Model file for the job. Use its own axes, mm. A direction names the side the tool comes from. Coordinates: 2 decimals unless noted, no trailing zeros. Order: outer loops, then holes, each group sorted by start corner. A loop starts at its lowest first (then second) coordinate and runs counter-clockwise, first axis right, second up.
from build123d import *

# Parameters (mm, degrees)
F1_DEPTH      = 152.4
F1_DEPTH_BACK = 152.4
F2_W          = 381.0055409819
F2_H          = 19.05
F2_W_2        = 381
F3_DEPTH      = 6.096
F4_W          = 381.0055409819
F4_H          = 19.05
F4_W_2        = 381
F5_DEPTH      = 6.096


# Not quite as in the source:
# - ends of sketch curves that miss each other by under 0.0002 mm in the source are joined


with BuildPart() as f1:
    # F0 (on Front) → F1 (new body, two sides)
    with BuildSketch(Plane.XZ) as f1_sk:
        Polygon((-533.4, -382.5126007106), (-381, -382.5126007106), (-381, -378.4719215088), (0, -378.4719215088), (0, -359.4219215088), (-381, -359.4219215088), (-381, -356.2469204928), (-381, -12.157774965), (-381, -8.982775981), (0.0055409819, -8.982775981), (0.0055409819, 10.067224019), (-381, 10.067224019), (-381, 13.242225035), (-381, 355.2765448173), (-381, 358.4515458333), (0.0055409819, 358.4515458333), (0.0055409819, 377.5015458333), (-381, 377.5015458333), (-381, 380.6765448173), (-533.4, 380.6765468493), align=None)
    extrude(amount=F1_DEPTH)
    extrude(f1_sk.sketch, amount=-F1_DEPTH_BACK)

    # F2 (on face) → F3 (cut)
    with BuildSketch(Plane(origin=(0, 152.4, 0), x_dir=(-1, 0, 0), z_dir=(0, 1, 0))):
        with Locations((190.4972295091, 367.9765458333)):
            Rectangle(F2_W, F2_H)
        with Locations((190.4972295091, 0.542224019)):
            Rectangle(F2_W, F2_H)
        with Locations((190.5, -368.9469215088)):
            Rectangle(F2_W_2, F2_H)
    extrude(amount=-F3_DEPTH, mode=Mode.SUBTRACT)

    # F4 (on face) → F5 (cut)
    with BuildSketch(Plane.XZ.offset(152.4)):
        with Locations((-190.4972295091, 0.542224019)):
            Rectangle(F4_W, F4_H)
        with Locations((-190.4972295091, 367.9765458333)):
            Rectangle(F4_W, F4_H)
        with Locations((-190.5, -368.9469215088)):
            Rectangle(F4_W_2, F4_H)
    extrude(amount=-F5_DEPTH, mode=Mode.SUBTRACT)


solid = f1.part
Q1. Cut at A-A, the plane x = -277.5. List the corners of the cut face in (y, z), plus the area to 3 significant figures.
Established:
outline: (-146.3, -378.47) - (146.3, -378.47) - (146.3, -359.42) - (-146.3, -359.42) - close; (-146.3, -8.98) - (146.3, -8.98) - (146.3, 10.07) - (-146.3, 10.07) - close; (-146.3, 358.45) - (146.3, 358.45) - (146.3, 377.5) - (-146.3, 377.5) - close
area: 16,700 mm2
Q2. Cut at C-C, the plane z = 302. List the corners of the cut face in (x, y), plus the area to 3 significant figures.
Established:
outline: (-533.4, -152.4) - (-381, -152.4) - (-381, 152.4) - (-533.4, 152.4) - close
area: 46,500 mm2
Q3. Cut at B-B, the plane y = -98.5. List the corners of the cut face in (x, z).
Established:
outline: (-533.4, -382.51) - (-381, -382.51) - (-381, -378.47) - (0, -378.47) - (0, -359.42) - (-381, -359.42) - (-381, -8.98) - (0.01, -8.98) - (0.01, 10.07) - (-381, 10.07) - (-381, 358.45) - (0.01, 358.45) - (0.01, 377.5) - (-381, 377.5) - (-381, 380.68) - (-533.4, 380.68) - close
Q4. Drop flat-ended pins along their axis: P1, Ø5.5, axis at x = -250.5, z = 372, coming from the +Y side; P2, Ø21, axis at x = -174.5, z = 369.5, coming from the -Y side; P3, Ø1, axis at x = -326, y = -16.5, coming from the +Z side. Give the stop position or say it passes through.
Established:
P1: stops at y = 146.3
P2: stops at y = -146.3
P3: stops at z = 377.5
Q5. Mould opens along Z. For faces 1 (the face through (0.006, -2, 0)), 2 (the face through (-193, -2, -378.472)), 3 (the face through (-193, -2, 358.452)), 4 (the face through (-188, -2, -359.422)) say: pulls with the +Z half, pulls with the -Z half, needs draft (parallel to the pull), parting line crosses it, or undercut.
Established:
face 1: needs draft
face 2: pulls with the -Z half
face 3: undercut
face 4: undercut
Q6. Which spindle directions (+Z, -Z, +X, -X, +Y, -Y) get a long thin tool onto all of the face, cutting with end or side? Do faces 5 (the face through (-188, -2, 10.067)), 6 (the face through (-193, -146.304, 368)), 7 (the face through (-188, -2, 377.502)), 8 (the face through (-188, 146.304, 1)). Say none if no direction does.
Established:
face 5: +X, +Y, -Y
face 6: +Z, -Z, +X, -Y
face 7: +Z, +X, +Y, -Y
face 8: +Z, -Z, +X, +Y
Q7. Probe line 1 (Z direction, x = -173, y = 99); line 2 (X direction, y = 48, z = -266). List the from-to ranges inside material, lowest first.
Established:
line 1: z = -378.47 to -359.42, -8.98 to 10.07, 358.45 to 377.5
line 2: x = -533.4 to -381
